Model file for the job. Use its own axes, mm. Coordinates: 2 decimals unless noted, no trailing zeros. Write each loop counter-clockwise with the first axis right and the second up, starting at its lowest first coordinate (ties: lowest second). Pieces come first, ordered by that corner, then holes. Notation, with made-up numbers: M -1.5,-12 L 12.5,-12 A12 cw 12.5,-4 Z; hole C -14,83.25 d10. An arc over 180 degrees is marked long. One line per question, with ' | ' between items. Start each with the question number.
(1) Two-plate mould, pull along Y, no slides. Class faces 1 (the face through (-43, -9.096, 1)), 2 (the face through (-25.493, 17, 1)), 3 (the face through (-30.028, 34.504, 0.986)): +Y half, -Y half, draft (parallel to the pull), parting line (faces both ways), or undercut.
(2) Cut at A-A (y = 32). Write the cut outline in (x, z).
(3) Flat gauge pin, fed straight in: pin 1 Ø4 at (x, y) = (-28.77, 18.93) entering from -Z. Where does the tip first touch, or does it go through?
(4) Cut at C-C (z = 1.15). Write the cut outline in (x, y).
(5) Wall check: probe 1 along X at (y, z) = (19.5, 1.7); probe 2 along X at (y, z) = (20, 0.9); probe 3 along X at (y, z) = (35, 0.15). Give the ranges that are in metal, low to high.
(6) Cut at B-B (x = -50). Write the cut outline in (y, z).
Autodesk Inventor part; units mm, degrees
ref_plane "YZ Plane" through (0, 0, 0) normal (1, 0, 0) x (0, 1, 0)
ref_plane "XZ Plane" through (0, 0, 0) normal (0, 1, 0) x (-1, 0, 0)
ref_plane "XY Plane" through (0, 0, 0) normal (0, 0, 1) x (1, 0, 0)
sketch "Sketch2" plane through (0, 0, 0) normal (0, 0, 1) x (1, 0, 0)
  circle A0 centre (-42.2678, 29.4289) radius 13.25
  line L0 (-25.4928, 43.2039) -> (-59.0428, 43.2039)
  line L1 (-25.4928, -9.0961) -> (-25.4928, 43.2039)
  line L2 (-59.0428, 43.2039) -> (-59.0428, -9.0961)
  line L3 (-59.0428, -9.0961) -> (-25.4928, -9.0961)
  line L4 (-25.4928, -9.0961) -> (-25.4928, 43.2039)
  line L5 (-59.0428, -9.0961) -> (-25.4928, -9.0961)
  circle A1 centre (-55.7678, 18.9289) radius 1.5
  circle A2 centre (-28.7678, 18.9289) radius 1.5
  point P0 (0, 0)
  point P1 (-25.4928, -10.1461)
  dimension "d10" = 26.5
  dimension "d11" = 13.775
  dimension "d12" = 16.775
  dimension "d14" = 3
  dimension "d15" = 10.5
  dimension "d16" = 3
  dimension "d17" = 27
  dimension "d18" = 10.5
  dimension "d19" = 3.275
  dimension "d22" = 52.3
extrude "Extrusion1" add sketch "Sketch2" along normal blind 2
properties part number "Motor_Cover_2"
Filled in:
1) face 1: -Y half | face 2: draft | face 3: undercut
2) outline: M -59.04,0 L -55.27,0 L -55.27,2 L -59.04,2 Z; M -29.27,0 L -25.49,0 L -25.49,2 L -29.27,2 Z
3) pin 1: z = 0
4) outline: M -59.04,-9.1 L -25.49,-9.1 L -25.49,43.2 L -59.04,43.2 Z; hole C -55.77,18.93 d3; hole C -42.27,29.43 d26.5; hole C -28.77,18.93 d3
5) probe 1: -59.04 to -57.15, -54.38 to -51.04, -33.49 to -30.15, -27.38 to -25.49 | probe 2: -59.04 to -56.82, -54.72 to -51.58, -32.96 to -29.82, -27.72 to -25.49 | probe 3: -59.04 to -54.29, -30.25 to -25.49
6) outline: M -9.1,0 L 18.67,0 L 18.67,2 L -9.1,2 Z; M 40.19,0 L 43.2,0 L 43.2,2 L 40.19,2 Z
